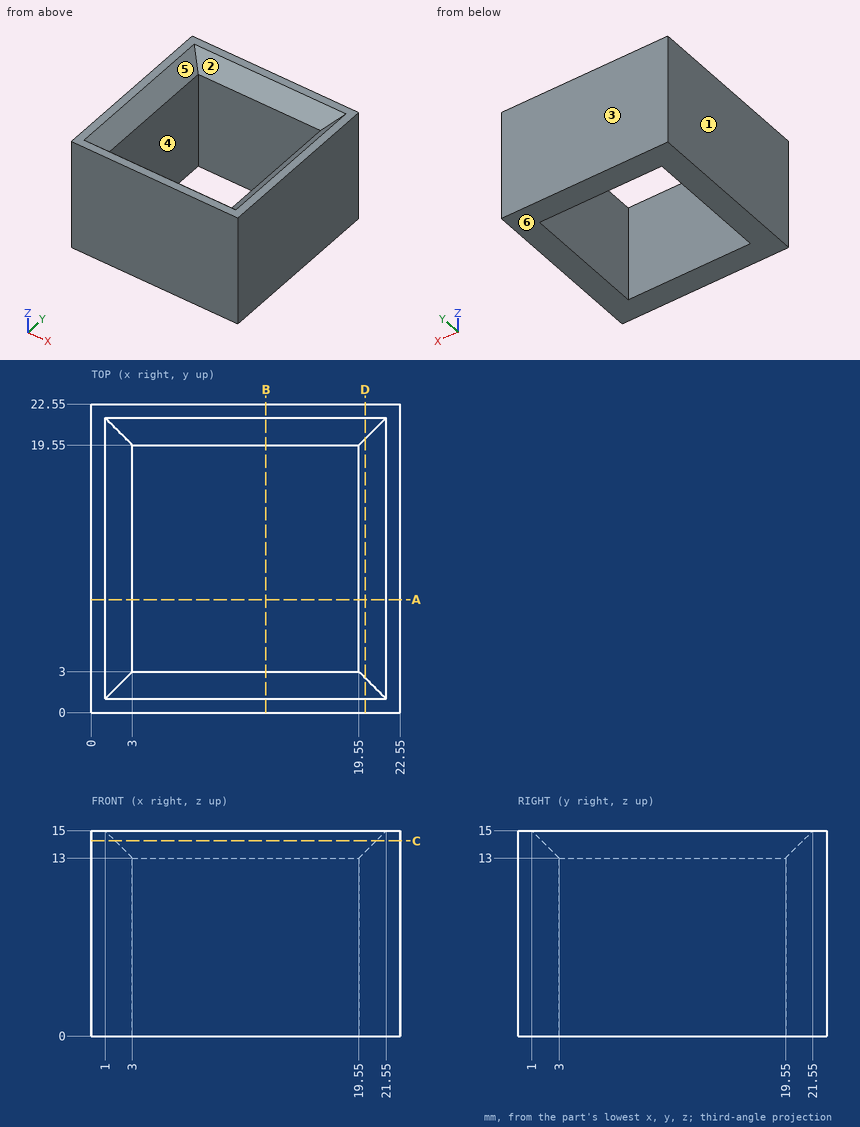
Study the drawing (mm; zero at the part's minimum x, y, z) and answer. A direction names the side the tool comes from. Coordinates: 2 decimals unless noted, no trailing zeros. Write each loop counter-clockwise with the first axis right and the second up, starting at its lowest first coordinate (ties: lowest second). Pieces come first, ordered by that corner, then holes. Notation, with made-up numbers: (-17, 33) - (-9, 33) arc R14 ccw to (-9, 38) - close; hole circle Ø9 at (54.5, 4). An arc over 180 degrees is marked (long way). One line per question, with ' | ' between items.
1) For the marked faces 4, 5 and 6, determine the directions among +Z, -Z, +X, -X, +Y, -Y from which every point of the face is accessible in a straight line to the end or side of a thin tool.
Checks:
face 4: +Z, -Z | face 5: +Z | face 6: -Z, +X, -X, +Y, -Y
2) Consider probe 1 along X at (y, z) = (9, 6); probe 2 along Z at (x, y) = (20, 6). Determine where each line is inside the solid, lowest interval first. Write a range as [from, to].
Checks:
probe 1: [0, 3], [19.55, 22.55] | probe 2: [0, 13.45]
3) Find section A-A, the plane y = 8.25. Determine the outline of the cut face in (x, z), and give its area (3 significant figures).
Checks:
outline: (0, 0) - (3, 0) - (3, 13) - (1, 15) - (0, 15) - close; (19.55, 0) - (22.55, 0) - (22.55, 15) - (21.55, 15) - (19.55, 13) - close | area: 86.0 mm2
4) Find section D-D, the plane x = 20. Determine the outline of the cut face in (y, z), and give its area (3 significant figures).
Checks:
outline: (0, 0) - (22.55, 0) - (22.55, 15) - (21.55, 15) - (20, 13.45) - (2.55, 13.45) - (1, 15) - (0, 15) - close | area: 309 mm2
5) Find section C-C, the plane z = 14.25. Determine the outline of the cut face in (x, y), and give its area (3 significant figures).
Checks:
outline: (0, 0) - (22.55, 0) - (22.55, 22.55) - (0, 22.55) - close; hole (1.75, 1.75) - (20.8, 1.75) - (20.8, 20.8) - (1.75, 20.8) - close | area: 146 mm2
6) The mould has two halves that part along Y. Classify the marked faces 1, 2 and 3: +Y half, -Y half, draft (parallel to the pull), parting line (faces both ways), or undercut.
Checks:
face 1: draft | face 2: undercut | face 3: +Y half
